Read the model definition and answer for the solid it produces. Units are mm, in the model's axes. A direction names the side the tool comes from. Coordinates: 2 decimals unless noted, no trailing zeros. Loops run counter-clockwise (first coordinate to the right, second up) from the corner with the lowest first, then second, coordinate; pieces in that order, holes last.
from build123d import *

# Parameters (mm, degrees)
SKETCH1_W           = 70
SKETCH1_H           = 70
BOSS_EXTRUDE1_DEPTH = 3
SKETCH2_R           = 14.255
CUT_EXTRUDE1_DEPTH  = 3


with BuildPart() as part:
    # Sketch1 → Boss-Extrude1 (new body)
    with BuildSketch(Plane(origin=(0, 0, 0), x_dir=(1, 0, 0), z_dir=(0, 1, 0))):
        with Locations((35, 35)):
            Rectangle(SKETCH1_W, SKETCH1_H)
    extrude(amount=BOSS_EXTRUDE1_DEPTH)

    # Sketch2 → Cut-Extrude1 (cut)
    with BuildSketch(Plane(origin=(0, 3, 0), x_dir=(1, 0, 0), z_dir=(0, 1, 0))):
        with Locations((35.251413305, 34.802601327)):
            Circle(SKETCH2_R)
        with BuildLine():
            Line((10.75, 63.008410324), (10.75, 6.991589676))
            ThreePointArc((10.75, 6.991589676), (8, 4.241589676), (5.25, 6.991589676))
            Line((5.25, 6.991589676), (5.25, 63.008410324))
            ThreePointArc((5.25, 63.008410324), (8, 65.758410324), (10.75, 63.008410324))
        make_face()
        with BuildLine():
            Line((64.75, 63.008410324), (64.75, 6.991589676))
            ThreePointArc((64.75, 6.991589676), (62, 4.241589676), (59.25, 6.991589676))
            Line((59.25, 6.991589676), (59.25, 63.008410324))
            ThreePointArc((59.25, 63.008410324), (62, 65.758410324), (64.75, 63.008410324))
        make_face()
    extrude(amount=-CUT_EXTRUDE1_DEPTH, mode=Mode.SUBTRACT)


solid = part.part
Q1. Which of the six approach directions +Z, -Z, +X, -X, +Y, -Y give full straight-line access (tool end or side, diameter ignored) to faces 1 (the face through (64.75, 2, -35)), 2 (the face through (0, 1, -35))?
Findings below:
face 1: +Y, -Y
face 2: +Z, -Z, -X, +Y, -Y
Q2. A cutting plane is placed at D-D (y = 1.5). Give the vertices of the cut face in (x, z) (3 decimals).
Findings below:
outline: (0, -70) - (70, -70) - (70, 0) - (0, 0) - close; hole (5.25, -63.008) arc R2.75 ccw to (10.75, -63.008) - (10.75, -6.992) arc R2.75 ccw to (5.25, -6.992) - close; hole circle Ø28.51 at (35.251, -34.803); hole (59.25, -63.008) arc R2.75 ccw to (64.75, -63.008) - (64.75, -6.992) arc R2.75 ccw to (59.25, -6.992) - close
Q3. A cutting plane is placed at C-C (z = -41). Give the vertices of the cut face in (x, y).
Findings below:
outline: (0, 0) - (5.25, 0) - (5.25, 3) - (0, 3) - close; (10.75, 0) - (22.41, 0) - (22.41, 3) - (10.75, 3) - close; (48.09, 0) - (59.25, 0) - (59.25, 3) - (48.09, 3) - close; (64.75, 0) - (70, 0) - (70, 3) - (64.75, 3) - close
Q4. Determine the mould class of faces 3 (the face through (35, 1, -70)), 4 (the face through (70, 1, -35)), 5 (the face through (61.94, 1.521, -65.758)) for opening direction Z: +Z half, -Z half, draft (parallel to the pull), parting line (faces both ways), or undercut.
Findings below:
face 3: -Z half
face 4: draft
face 5: undercut
Q5. A cutting plane is placed at A-A (x = 8). Give the vertices of the cut face in (y, z), then the cut area to 3 significant figures.
Findings below:
outline: (0, -70) - (3, -70) - (3, -65.76) - (0, -65.76) - close; (0, -4.24) - (3, -4.24) - (3, 0) - (0, 0) - close
area: 25.4 mm2
Q6. Straight lines are drawn through the part: probe 1 along X at (y, z) = (2.05, -20); probe 2 along X at (y, z) = (0.65, -44); probe 3 along X at (y, z) = (1.45, -31). For each, find the intervals that lie inside material, in ascending order.
Findings below:
probe 1: x = 0 to 5.25, 10.75 to 59.25, 64.75 to 70
probe 2: x = 0 to 5.25, 10.75 to 24.36, 46.14 to 59.25, 64.75 to 70
probe 3: x = 0 to 5.25, 10.75 to 21.51, 48.99 to 59.25, 64.75 to 70
Q7. A cutting plane is placed at B-B (z = -60.5). Give the vertices of the cut face in (x, y), then the cut area to 3 significant figures.
Findings below:
outline: (0, 0) - (5.25, 0) - (5.25, 3) - (0, 3) - close; (10.75, 0) - (59.25, 0) - (59.25, 3) - (10.75, 3) - close; (64.75, 0) - (70, 0) - (70, 3) - (64.75, 3) - close
area: 177 mm2
Q8. A flat-ended cylindrical pin translates along its axis: pin 1 Ø17 at (x, z) = (35.25, -34.8) entering from -Y. Find the tip coordinate at first contact, or state that the pin passes through.
Findings below:
pin 1: passes through
